The drawing under review shows one solid part. Ordinate dimensions are in mm from its lowest x, y, z. A direction names the side the tool comes from. Coordinates: 2 decimals unless noted, no trailing zeros. Write each loop counter-clockwise with the first axis right and the second up, starting at its lowest first coordinate (ties: lowest second). Pieces come first, ordered by that corner, then holes.
Q1. To check wall thickness, follow probe 1 along Z at (x, y) = (43.25, 10); probe 2 along X at (y, z) = (9.75, 40); probe 3 along Y at (x, z) = (39, 44). State the ranges of each line that lie inside material, in increasing order.
Q2. Machinability: for the marked faces 4, 5, 6 and 7, which of the approach directions +Z, -Z, +X, -X, +Y, -Y give a long, thin tool a straight path to every point of the face, cutting with its end or side? Answer none if there is none.
Q3. The part is to be moulded in two halves that separate along X. For the marked faces 1, 2 and 3, say which applies: +X half, -X half, draft (parallel to the pull), parting line (faces both ways), or undercut.
Q4. Add section D-D, the plane x = 8. Give the boundary of the cut face in (y, z), plus the area to 3 significant figures.
Q5. Add section B-B, the plane y = 10. Give the number of separate pieces and of enclosed holes in the cut face, plus the area to 3 significant figures.
Q6. Add section A-A, the plane z = 44.05. Give the boundary of the cut face in (x, y), plus the area to 3 significant figures.
Q7. Clearance check with flat-ended pins moving along their axes: pin 1 Ø6 at (y, z) = (5, 31.5) entering from +X; pin 2 Ø6 at (y, z) = (11.5, 32.5) entering from -X; pin 3 Ø3 at (x, y) = (22, 16.5) entering from +Z. State where each tip first meets the part, or that it passes through.
Q8. Add section C-C, the plane z = 14. Give the boundary of the cut face in (x, y).
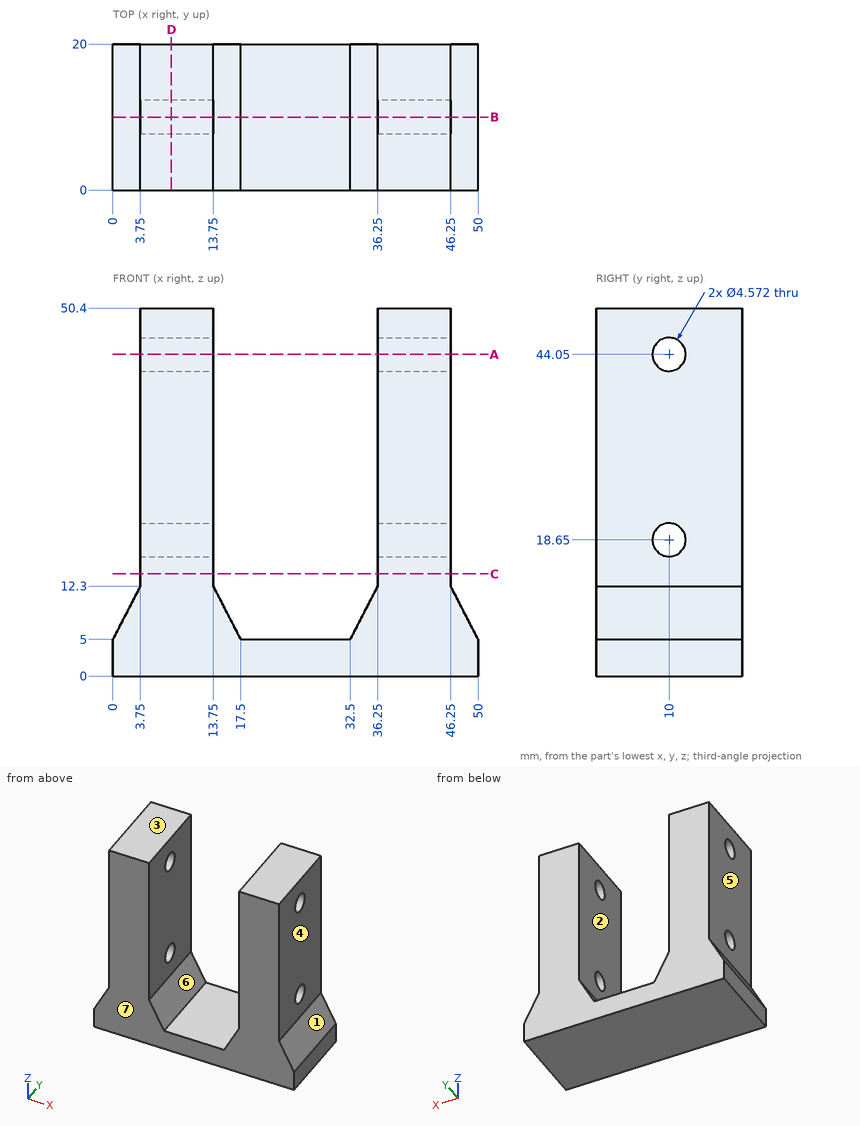
Here are the results:
1. probe 1: z = 0 to 16.36, 20.94 to 41.76, 46.34 to 50.4
1. probe 2: x = 3.75 to 13.75, 36.25 to 46.25
1. probe 3: y = 0 to 7.71, 12.29 to 20
2. face 4: +Z, +X, +Y, -Y
2. face 5: +Z, -X, +Y, -Y
2. face 6: +Z, +Y, -Y
2. face 7: +Z, -Z, +X, -X, -Y
3. face 1: +X half
3. face 2: undercut
3. face 3: draft
4. outline: (0, 0) - (20, 0) - (20, 50.4) - (0, 50.4) - close; hole circle Ø4.57 at (10, 18.65); hole circle Ø4.57 at (10, 44.05)
4. area: 975 mm2
5. separate pieces: 5
5. enclosed holes: 0
5. area: 1,030 mm2
6. outline: (3.75, 0) - (13.75, 0) - (13.75, 7.71) - (3.75, 7.71) - close; (3.75, 12.29) - (13.75, 12.29) - (13.75, 20) - (3.75, 20) - close; (36.25, 0) - (46.25, 0) - (46.25, 7.71) - (36.25, 7.71) - close; (36.25, 12.29) - (46.25, 12.29) - (46.25, 20) - (36.25, 20) - close
6. area: 309 mm2
7. pin 1: stops at x = 46.25
7. pin 2: stops at x = 3.75
7. pin 3: stops at z = 5
8. outline: (3.75, 0) - (13.75, 0) - (13.75, 20) - (3.75, 20) - close; (36.25, 0) - (46.25, 0) - (46.25, 20) - (36.25, 20) - close
